For this review, take the finished solid that the model builds, in its own axes (mm). A direction names the side the tool comes from. Round coordinates to 2 decimals unless told otherwise and drop trailing zeros. Order: outer loops, then holes, each group sorted by start corner. A loop starts at its lowest first (then second) coordinate and runs counter-clockwise, first axis right, second up. Notation, with made-up numbers: (49, -38) - (74, -38) arc R18 ccw to (74, -29) - close; hole circle Ø11 at (22, -16.75). An arc over 180 degrees is marked (long way). One line per item, written item: value.
```python
from build123d import *

# Parameters (mm, degrees)
SKETCH1_W           = 350
SKETCH1_H           = 350
SKETCH1_W_2         = 310
SKETCH1_H_2         = 59
SKETCH1_H_3         = 149
SKETCH1_H_4         = 62
BOSS_EXTRUDE1_DEPTH = 20
SKETCH2_W           = 350
SKETCH2_H           = 40
BOSS_EXTRUDE2_DEPTH = 5
SKETCH3_W           = 20
SKETCH3_H           = 20
BOSS_EXTRUDE4_DEPTH = 150
SKETCH4_R           = 4
CUT_EXTRUDE1_DEPTH  = 339.914592404
SKETCH5_R           = 4
CUT_EXTRUDE2_DEPTH  = 351.735228342
SKETCH6_R           = 4
CUT_EXTRUDE3_DEPTH  = 339.914592404


with BuildPart() as part:
    # Sketch1 → Boss-Extrude1 (new body)
    with BuildSketch(Plane.XY):
        with Locations((-0.376590763, -86.214953271)):
            Rectangle(SKETCH1_W, SKETCH1_H)
        with Locations((-0.376590763, -128.45502947)):
            Rectangle(SKETCH1_W_2, SKETCH1_H_2, mode=Mode.SUBTRACT)
        with Locations((-0.376590763, -4.45502947)):
            Rectangle(SKETCH1_W_2, SKETCH1_H_3, mode=Mode.SUBTRACT)
        with Locations((-0.376590763, -208.95502947)):
            Rectangle(SKETCH1_W_2, SKETCH1_H_4, mode=Mode.SUBTRACT)
    extrude(amount=BOSS_EXTRUDE1_DEPTH)

    # Sketch2 → Boss-Extrude2 (add)
    with BuildSketch(Plane.XY.offset(20)):
        with Locations((-0.376590763, -19.95502947)):
            Rectangle(SKETCH2_W, SKETCH2_H)
    extrude(amount=BOSS_EXTRUDE2_DEPTH)

    # Sketch3 → Boss-Extrude4 (add)
    with BuildSketch(Plane.XY.offset(25)):
        with Locations((-70.876590763, -19.95502947)):
            Rectangle(SKETCH3_W, SKETCH3_H)
        with Locations((70.123409237, -19.95502947)):
            Rectangle(SKETCH3_W, SKETCH3_H)
    extrude(amount=BOSS_EXTRUDE4_DEPTH)

    # Sketch4 → Cut-Extrude1 (cut, through all)
    with BuildSketch(Plane.XZ.offset(29.95502947)):
        with Locations(Location((-70.876590763, 135, 0), (0, 0, 270))):
            Circle(SKETCH4_R)
        with Locations(Location((-70.876590763, 85, 0), (0, 0, 270))):
            Circle(SKETCH4_R)
        with Locations(Location((70.123409237, 135, 0), (0, 0, 270))):
            Circle(SKETCH4_R)
        with Locations(Location((70.123409237, 85, 0), (0, 0, 270))):
            Circle(SKETCH4_R)
    extrude(amount=-CUT_EXTRUDE1_DEPTH, mode=Mode.SUBTRACT)

    # Sketch5 → Cut-Extrude2 (cut, through all)
    with BuildSketch(Plane.XY.offset(20)):
        with Locations((-38.918433774, -87.591447664)):
            Circle(SKETCH5_R)
        with Locations((-12.765040303, -87.591447664)):
            Circle(SKETCH5_R)
        with Locations((14.076600366, -87.591447664)):
            Circle(SKETCH5_R)
        with Locations((38.165252248, -87.591447664)):
            Circle(SKETCH5_R)
        with Locations((62.25390413, -87.591447664)):
            Circle(SKETCH5_R)
        with Locations((62.25390413, -168.804616866)):
            Circle(SKETCH5_R)
        with Locations((38.165252248, -168.804616866)):
            Circle(SKETCH5_R)
        with Locations((14.076600366, -168.804616866)):
            Circle(SKETCH5_R)
        with Locations((-12.765040303, -168.804616866)):
            Circle(SKETCH5_R)
        with Locations((-38.918433774, -168.804616866)):
            Circle(SKETCH5_R)
    extrude(amount=-CUT_EXTRUDE2_DEPTH, mode=Mode.SUBTRACT)

    # Sketch6 → Cut-Extrude3 (cut, through all)
    with BuildSketch(Plane.XZ.offset(29.95502947)):
        with Locations(Location((-70.876590763, 110, 0), (0, 0, 270))):
            Circle(SKETCH6_R)
        with Locations(Location((70.285399923, 110, 0), (0, 0, 270))):
            Circle(SKETCH6_R)
    extrude(amount=-CUT_EXTRUDE3_DEPTH, mode=Mode.SUBTRACT)


solid = part.part
```
Item 1: For P1, Ø13, axis at x = 38.17, y = -168.8, coming from the +Z side; P2, Ø4, axis at x = -81, z = 23.5, coming from the +Y side (3 decimals); P3, Ø6, axis at y = -19, z = 101, coming from the -X side, all flat-tipped, find the tip position at first contact; note any pin that passes through.
Returned:
P1: z = 20
P2: y = 0.045
P3: x = -80.88
Item 2: Take a section at B-B (y = -201.5). Write out the cut boundary in (x, z), plus the area to 3 significant figures.
Returned:
outline: (-175.38, 0) - (-155.38, 0) - (-155.38, 20) - (-175.38, 20) - close; (154.62, 0) - (174.62, 0) - (174.62, 20) - (154.62, 20) - close
area: 800 mm^2
Item 3: Wall thickness on line 1 (Y direction, x = 116, z = 19.5); line 2 (X direction, y = -18, z = 85); line 3 (X direction, y = -21, z = 110): over which ranges is each line inside the solid? List them lowest first.
Returned:
line 1: -261.21 to -239.96, -177.96 to -157.96, -98.96 to -78.96, 70.04 to 88.79
line 2: -80.88 to -74.88, -66.88 to -60.88, 60.12 to 66.12, 74.12 to 80.12
line 3: -80.88 to -74.88, -66.88 to -60.88, 60.12 to 66.29, 74.29 to 80.12
Item 4: Machinability: for faces 1 (the flat face through (-80.877, -20, 99)), 2 (the flat face through (70, -29.955, 99)), 3 (the flat face through (-3, -20, 20)), 4 (the flat face through (-155.377, -209, 10)), 5 (the flat face through (-60.877, -20, 99)), which of the approach directions +Z, -Z, +X, -X, +Y, -Y give a long, thin tool a straight path to every point of the face, cutting with its end or side? Answer none if there is none.
Returned:
face 1: +Z, -X, +Y, -Y
face 2: +Z, +X, -X, -Y
face 3: -Z
face 4: +Z, -Z
face 5: +Z, +Y, -Y
Item 5: Take a section at A-A (z = 124.5). Write out the cut boundary in (x, y).
Returned:
outline: (-80.88, -29.96) - (-60.88, -29.96) - (-60.88, -9.96) - (-80.88, -9.96) - close; (60.12, -29.96) - (80.12, -29.96) - (80.12, -9.96) - (60.12, -9.96) - close
Item 6: Take a section at C-C (y = -16). Write out the cut boundary in (x, z).
Returned:
outline: (-175.38, 0) - (-155.38, 0) - (-155.38, 20) - (154.62, 20) - (154.62, 0) - (174.62, 0) - (174.62, 25) - (80.12, 25) - (80.12, 175) - (60.12, 175) - (60.12, 25) - (-60.88, 25) - (-60.88, 175) - (-80.88, 175) - (-80.88, 25) - (-175.38, 25) - close; hole circle Ø8 at (-70.88, 85); hole circle Ø8 at (-70.88, 110); hole circle Ø8 at (-70.88, 135); hole circle Ø8 at (70.12, 85); hole circle Ø8 at (70.12, 135); hole circle Ø8 at (70.29, 110)
Item 7: The part is to be moulded in two halves that separate along X. For faces 6 (the flat face through (-71, -29.955, 99)), 7 (the flat face through (-175.377, -89, 10)), 8 (the cylindrical face through (-13.29, -164.84, 10.14)), say which applies: +X half, -X half, draft (parallel to the pull), parting line (faces both ways), or undercut.
Returned:
face 6: draft
face 7: -X half
face 8: undercut
